from build123d import *

# Parameters (mm, degrees)
SKETCH1_W           = 20
SKETCH1_H           = 32
SKETCH1_R           = 1.5
BOSS_EXTRUDE1_DEPTH = 10
SKETCH3_R           = 12.5
BOSS_EXTRUDE2_DEPTH = 200
SKETCH4_OUTSIDE_W   = 73.936
SKETCH4_OUTSIDE_H   = 73.936
SKETCH4_OUTSIDE_W_2 = 15
SKETCH4_OUTSIDE_H_2 = 15
CUT_EXTRUDE1_DEPTH  = 10
SKETCH5_R           = 1.5
CUT_EXTRUDE2_DEPTH  = 234.195733237


with BuildPart() as part:
    # Sketch1 → Boss-Extrude1 (new, symmetric)
    with BuildSketch(Plane.XY):
        with Locations((0, 16)):
            Rectangle(SKETCH1_W, SKETCH1_H)
        with Locations((0, 5)):
            Circle(SKETCH1_R, mode=Mode.SUBTRACT)
        with Locations((0, 25)):
            Circle(SKETCH1_R, mode=Mode.SUBTRACT)
    extrude(amount=BOSS_EXTRUDE1_DEPTH, both=True)

    # Sketch3 → Boss-Extrude2 (add)
    with BuildSketch(Plane(origin=(0, 32, 0), x_dir=(1, 0, 0), z_dir=(0, 1, 0))):
        with Locations(Location((0, 0, 0), (0, 0, 53.130102354))):
            Circle(SKETCH3_R)
    extrude(amount=BOSS_EXTRUDE2_DEPTH)

    # Sketch4 outside → Cut-Extrude1 (cut)
    with BuildSketch(Plane(origin=(0, 232, 0), x_dir=(1, 0, 0), z_dir=(0, 1, 0))):
        Rectangle(SKETCH4_OUTSIDE_W, SKETCH4_OUTSIDE_H)
        Rectangle(SKETCH4_OUTSIDE_W_2, SKETCH4_OUTSIDE_H_2, mode=Mode.SUBTRACT)
    extrude(amount=-CUT_EXTRUDE1_DEPTH, mode=Mode.SUBTRACT)

    # Sketch5 → Cut-Extrude2 (cut, through all)
    with BuildSketch(Plane.XY.offset(7.5)):
        with Locations((0, 227)):
            Circle(SKETCH5_R)
    extrude(amount=-CUT_EXTRUDE2_DEPTH, mode=Mode.SUBTRACT)


solid = part.part
Read the model definition and answer for the solid it produces. Units are mm, in the model's axes. A direction names the side the tool comes from. Give positions to 0.01 mm unless a question says otherwise; leave off trailing zeros. Write each loop counter-clockwise with the first axis right and the second up, starting at its lowest first coordinate (ties: lowest second). Pieces come first, ordered by that corner, then holes. Notation, with made-up numbers: (63.5, 31) - (114.5, 31) arc R31 cw to (114.5, 68) - close; hole circle Ø5 at (-28.5, 76.25). An arc over 180 degrees is marked (long way). Answer in a Markdown table with one row per item. Add a question column.
Item 1: Section B-B, the plane y = 202 is taken. Write down the section's boundary in (x, z), and give its area (3 significant figures).
Item 2: A tool of negligible diameter and unlimited length cuts with its end or side. For faces 1 (the face through (0, 16, -10)), 2 (the face through (-2, 227, -7.5)), 3 (the face through (-2, 227, 7.5)), 4 (the face through (-7.5, 227, 0)), 5 (the face through (0, 16, 10)), from which of +Z, -Z, +X, -X, +Y, -Y can it reach the whole face along a straight path? Write none if from no direction.
Item 3: Find the intervals of material crossed by L1, parallel to Y at x = 0, z = 4.5; L2, parallel to Y at x = -0.75, z = -4; L3, parallel to X at y = 163.5, z = -1, in increasing order.
Item 4: Section C-C, the plane x = -4.5 is taken. Write down the section's boundary in (y, z), and give its area (3 significant figures).
Item 5: Section A-A, the plane z = 0 is taken. Write down the section's boundary in (x, y), and give its area (3 significant figures).
Item 6: Flat-ended cylindrical pins translate along their axes: P1, Ø6, axis at y = 42.5, z = -1.5, coming from the +X side; P2, Ø8, axis at x = 0.5, y = 228.5, coming from the -Z side; P3, Ø3, axis at x = 8.5, y = 79.5, coming from the -Z side; P4, Ø1.5, axis at x = 9, z = 8.5, coming from the +Y side. Find the tip coordinate at first contact, or state that the pin passes through.
Recorded:
| question | item | result |
|---|---|---|
| 1 | outline | circle Ø25 at (0, 0) |
| 1 | area | 491 mm2 |
| 2 | face 1 | -Z, +X, -X, -Y |
| 2 | face 2 | -Z, +X, -X, +Y |
| 2 | face 3 | +Z, +X, -X, +Y |
| 2 | face 4 | +Z, -Z, -X, +Y |
| 2 | face 5 | +Z, +X, -X, -Y |
| 3 | L1 | y = 0 to 3.5, 6.5 to 23.5, 26.5 to 225.5, 228.5 to 232 |
| 3 | L2 | y = 0 to 3.7, 6.3 to 23.7, 26.3 to 225.7, 228.3 to 232 |
| 3 | L3 | x = -12.46 to 12.46 |
| 4 | outline | (0, -10) - (32, -10) - (32, -11.66) - (222, -11.66) - (222, -7.5) - (232, -7.5) - (232, 7.5) - (222, 7.5) - (222, 11.66) - (32, 11.66) - (32, 10) - (0, 10) - close |
| 4 | area | 5,220 mm2 |
| 5 | outline | (-12.5, 32) - (-10, 32) - (-10, 0) - (10, 0) - (10, 32) - (12.5, 32) - (12.5, 222) - (7.5, 222) - (7.5, 232) - (-7.5, 232) - (-7.5, 222) - (-12.5, 222) - close; hole circle Ø3 at (0, 5); hole circle Ø3 at (0, 25); hole circle Ø3 at (0, 227) |
| 5 | area | 5,520 mm2 |
| 6 | P1 | stops at x = 12.5 |
| 6 | P2 | stops at z = -7.5 |
| 6 | P3 | stops at z = -10.36 |
| 6 | P4 | stops at y = 222 |
